The listing builds one solid part. Answer for the finished solid, in the listing's coordinates (mm). A direction names the side the tool comes from. Round coordinates to 2 decimals unless told otherwise and drop trailing zeros. Order: outer loops, then holes, each group sorted by start corner. A loop starts at its lowest first (then second) coordinate and runs counter-clockwise, first axis right, second up. Notation, with made-up numbers: (-17, 28) -> (21, 28) arc R17 ccw to (21, 51) -> close; hole circle Ø5 at (80.25, 9). An arc over 180 degrees is marked (long way). Return JSON: item names as keys, results as strings. Group by question number.
(1) The part is cut by section C-C (z = 87). Determine the outline of the cut face in (x, y).
(2) Determine the mould class of faces 1 (the face through (-2.75, -507.18, 127.6)), 2 (the face through (-349.122, -991.417, 399.36)), 3 (the face through (-300, -1060, 390)) for opening direction X: +X half, -X half, draft (parallel to the pull), parting line (faces both ways), or undercut.
(3) This flat-tipped pin is pushed along its axis until it touches: pin 1 (3 mm diameter, centred on x = -294, z = 213.5, fed in from +Y). Where does it stop, or does it pass through?
(4) The part is cut by section A-A (x = -300). Determine the outline of the cut face in (y, z), plus the area to 3 significant figures.
(5) Which of the six approach directions +Z, -Z, +X, -X, +Y, -Y give full straight-line access (tool end or side, diameter ignored) to faces 4 (the face through (-412.688, -999.442, 301.438)), 5 (the face through (0, 0, 0)), 6 (the face through (-287.408, -1032.237, 391.653))?
(6) The part is cut by section B-B (y = -317.5). Determine the outline of the cut face in (x, z), plus the area to 3 significant figures.
(7) The part is cut by section D-D (x = -400). Determine the outline of the cut face in (y, z).
from build123d import *

# Parameters (mm, degrees)
CROQUIS1_R              = 12.7
SALIENTE_EXTRUIR1_DEPTH = 50
CROQUIS2_R              = 12.7


with BuildPart() as part:
    # Croquis1 → Saliente-Extruir1 (new body)
    with BuildSketch(Plane.XY):
        Circle(CROQUIS1_R)
    extrude(amount=SALIENTE_EXTRUIR1_DEPTH)

    # Barrer1: sweep along a curve in space
    with BuildLine() as barrer1_path:
        Line((0, 0, 50), (0, 0, 140))
        Line((0, 0, 140), (0, -1000, 140))
        Line((0, -1000, 140), (0, -1000, 210))
        Line((0, -1000, 210), (-400, -1000, 210))
        Line((-400, -1000, 210), (-400, -1000, 390))
        Line((-400, -1000, 390), (-300, -1000, 390))
        Line((-300, -1000, 390), (-300, -1060, 390))
    # Croquis2 → Barrer1 (sweep)
    with BuildSketch(Plane.XY.offset(50)):
        Circle(CROQUIS2_R)
    sweep(path=barrer1_path.line, transition=Transition.RIGHT)


solid = part.part
Answer below:
{
 "1": {"outline": "circle Ø25.4 at (0, 0)"},
 "2": {"face 1": "parting line", "face 2": "undercut", "face 3": "draft"},
 "3": {"pin 1": "stops at y = -987.46"},
 "4": {"outline": "(-1060, 377.3) -> (-1000, 377.3) arc R12.7 ccw to (-1000, 402.7) -> (-1060, 402.7) -> close; circle Ø25.4 at (-1000, 210)", "area": "2,280 mm²"},
 "5": {"face 4": "none", "face 5": "-Z, +X, -X, +Y, -Y", "face 6": "-Y"},
 "6": {"outline": "circle Ø25.4 at (0, 140)", "area": "507 mm²"},
 "7": {"outline": "(-1012.7, 210) arc R12.7 ccw to (-987.3, 210) -> (-987.3, 390) arc R12.7 ccw to (-1012.7, 390) -> close"}
}
